```python
from build123d import *

# Parameters (mm, degrees)
SKETCH9_W                    = 200
SKETCH9_H                    = 30
BASE_FLANGE2_DEPTH           = 3
EDGE_FLANGE1_STRIP_W         = 18
EDGE_FLANGE1_STRIP_H         = 3
EDGE_FLANGE1_STRIP_CUT_DEPTH = 200
EDGE_FLANGE1_DEPTH           = 200
EDGE_FLANGE2_STRIP_W         = 18
EDGE_FLANGE2_STRIP_H         = 3
EDGE_FLANGE2_STRIP_CUT_DEPTH = 200
EDGE_FLANGE2_DEPTH           = 200
CUT_EXTRUDE1_START           = -3
CUT_EXTRUDE1_OUTLINE_R       = 4
CUT_EXTRUDE1_DEPTH           = 3
CUT_EXTRUDE1_START_2         = -100
CUT_EXTRUDE1_2_DEPTH         = 50
CUT_EXTRUDE1_START_3         = 50
CUT_EXTRUDE1_3_DEPTH         = 50
SKETCH19_R                   = 3
CUT_EXTRUDE2_DEPTH           = 3


# Read off the part's stored shape, not the designer's step: Cut-Extrude1
# Sheet-metal steps are written as plain solids
with BuildPart() as part:
    # Sketch9 → Base-Flange2 (new body)
    with BuildSketch(Plane(origin=(0, 0, 0), x_dir=(1, 0, 0), z_dir=(0, 1, 0))):
        with Locations((0, 15)):
            Rectangle(SKETCH9_W, SKETCH9_H)
    extrude(amount=-BASE_FLANGE2_DEPTH)

    # Edge-Flange1 strip (across the edge) → Edge-Flange1 strip cut (cut)
    with BuildSketch(Plane(origin=(100, -3, 0), x_dir=(0, 0, -1), z_dir=(-1, 0, 0))):
        with Locations((-6, -1.5)):
            Rectangle(EDGE_FLANGE1_STRIP_W, EDGE_FLANGE1_STRIP_H)
    extrude(amount=EDGE_FLANGE1_STRIP_CUT_DEPTH, mode=Mode.SUBTRACT)

    # Edge-Flange1 section (across the edge) → Edge-Flange1 (add)
    with BuildSketch(Plane(origin=(100, -3, 0), x_dir=(0, 0, -1), z_dir=(-1, 0, 0))):
        with BuildLine():
            Line((-3, 3), (-3, 35))
            Line((-3, 35), (0, 35))
            Line((0, 35), (0, 3))
            ThreePointArc((0, 3), (0.878679656, 0.878679656), (3, 0))
            Line((3, 0), (3, -3))
            ThreePointArc((3, -3), (-1.242640687, -1.242640687), (-3, 3))
        make_face()
    extrude(amount=EDGE_FLANGE1_DEPTH)

    # Edge-Flange2 strip (across the edge) → Edge-Flange2 strip cut (cut)
    with BuildSketch(Plane(origin=(-100, -38, 3), x_dir=(0, 1, 0), z_dir=(1, 0, 0))):
        with Locations((-6, -1.5)):
            Rectangle(EDGE_FLANGE2_STRIP_W, EDGE_FLANGE2_STRIP_H)
    extrude(amount=EDGE_FLANGE2_STRIP_CUT_DEPTH, mode=Mode.SUBTRACT)

    # Edge-Flange2 section (across the edge) → Edge-Flange2 (add)
    with BuildSketch(Plane(origin=(-100, -38, 3), x_dir=(0, 1, 0), z_dir=(1, 0, 0))):
        with BuildLine():
            Line((-3, 3), (-3, 70))
            Line((-3, 70), (0, 70))
            Line((0, 70), (0, 3))
            ThreePointArc((0, 3), (0.878679656, 0.878679656), (3, 0))
            Line((3, 0), (3, -3))
            ThreePointArc((3, -3), (-1.242640687, -1.242640687), (-3, 3))
        make_face()
    extrude(amount=EDGE_FLANGE2_DEPTH)

    # Cut-Extrude1 outline → Cut-Extrude1 (cut)
    with BuildSketch(Plane(origin=(0, -38, 0), x_dir=(1, 0, 0), z_dir=(0, 1, 0)).offset(CUT_EXTRUDE1_START)):
        with Locations((0, -25.63)):
            Circle(CUT_EXTRUDE1_OUTLINE_R)
    extrude(amount=CUT_EXTRUDE1_DEPTH, mode=Mode.SUBTRACT)

    # Cut-Extrude1 2 outline → Cut-Extrude1 2 (cut)
    with BuildSketch(Plane.YZ.offset(CUT_EXTRUDE1_START_2)):
        with BuildLine():
            ThreePointArc((-41, 6), (-40.795554958, 4.447085729), (-40.196152423, 3))
            Line((-40.196152423, 3), (-37.598076212, 4.5))
            ThreePointArc((-37.598076212, 4.5), (-37.897777479, 5.223542864), (-38, 6))
            Line((-38, 6), (-38, 73))
            Line((-38, 73), (-41, 73))
            Line((-41, 73), (-41, 6))
        make_face()
    extrude(amount=CUT_EXTRUDE1_2_DEPTH, mode=Mode.SUBTRACT)

    # Cut-Extrude1 3 outline → Cut-Extrude1 3 (cut)
    with BuildSketch(Plane.YZ.offset(CUT_EXTRUDE1_START_3)):
        with BuildLine():
            ThreePointArc((-41, 6), (-40.795554958, 4.447085729), (-40.196152423, 3))
            Line((-40.196152423, 3), (-37.598076212, 4.5))
            ThreePointArc((-37.598076212, 4.5), (-37.897777479, 5.223542864), (-38, 6))
            Line((-38, 6), (-38, 73))
            Line((-38, 73), (-41, 73))
            Line((-41, 73), (-41, 6))
        make_face()
    extrude(amount=CUT_EXTRUDE1_3_DEPTH, mode=Mode.SUBTRACT)

    # Sketch19 → Cut-Extrude2 (cut)
    with BuildSketch(Plane(origin=(0, 0, 0), x_dir=(1, 0, 0), z_dir=(0, 1, 0))):
        with Locations(Location((-90, 15, 0), (0, 0, 270))):
            Circle(SKETCH19_R)
        with Locations(Location((-50, 15, 0), (0, 0, 270))):
            Circle(SKETCH19_R)
        with Locations(Location((50, 15, 0), (0, 0, 270))):
            Circle(SKETCH19_R)
        with Locations(Location((90, 15, 0), (0, 0, 270))):
            Circle(SKETCH19_R)
    extrude(amount=-CUT_EXTRUDE2_DEPTH, mode=Mode.SUBTRACT)


solid = part.part
```
For this review, take the finished solid that the model builds, in its own axes (mm). A direction names the side the tool comes from. Give positions to 0.01 mm unless a question says otherwise; leave off trailing zeros. Write each loop counter-clockwise with the first axis right and the second up, starting at its lowest first coordinate (ties: lowest second). Pieces come first, ordered by that corner, then holes. Notation, with made-up numbers: M -29.5,38 L -3.5,38 A24 cw -3.5,61 Z; hole C 15.5,-39.5 d9. An arc over 180 degrees is marked long. One line per item, written item: value.
1) For faces 4 (the flat face through (-1, -3, -17)), 5 (the cylindrical face through (-47, -1, -15)), 6 (the flat face through (1, -20, 3)), list the 3-axis set-ups (+Z, -Z, +X, -X, +Y, -Y) from which the entire face can be reached by the end or side of a thin tool; tool diameter is ignored.
Results are:
face 4: -Z, +X, -X, -Y
face 5: +Y, -Y
face 6: +Z, +X, -X, +Y
2) Take a section at A-A, the plane z = 25.63. Write out the cut boundary in (x, y), then the cut area to 3 significant figures.
Results are:
outline: M -50,-41 L -4,-41 L -4,-38 L -50,-38 Z; M 4,-41 L 50,-41 L 50,-38 L 4,-38 Z
area: 276 mm²
3) Take a section at C-C, the plane x = -7. Write out the cut boundary in (y, z), then the cut area to 3 significant figures.
Results are:
outline: M -41,6 A6 ccw -35,0 L -6,0 A3 cw -3,-3 L -3,-30 L 0,-30 L 0,-3 A6 ccw -6,3 L -35,3 A3 cw -38,6 L -38,73 L -41,73 Z
area: 411 mm²
4) For P1, Ø8, axis at x = 50, z = -15, coming from the -Y side; P2, Ø1, axis at y = -39, z = 24, coming from the +X side; P3, Ø8.5, axis at x = 36, y = -26.5, coming from the +Z side; P4, Ø5, axis at x = -50, z = -15, coming from the -Y side, all flat-tipped, find the tip position at first contact; note any pin that passes through.
Results are:
P1: stops at y = -3
P2: stops at x = 50
P3: stops at z = 3
P4: passes through
5) For line 1 (X direction, y = -1.45, z = -15); line 2 (Z direction, x = -82, y = -32.5); line 3 (Y direction, x = -39.5, z = -12.5), list the stretches that pass through material, from the lowest coordinate up. Write a range as from..to.
Results are:
line 1: x = -100..-93, -87..-53, -47..47, 53..87, 93..100
line 2: z = 0..3
line 3: y = -3..0
6) Take a section at B-B, the plane x = 90. Write out the cut boundary in (y, z).
Results are:
outline: M -40.2,3 A6 ccw -35,0 L -6,0 A3 cw -3,-3 L -3,-12 L 0,-12 L 0,-3 A6 ccw -6,3 L -35,3 A3 cw -37.6,4.5 Z; M -3,-30 L 0,-30 L 0,-18 L -3,-18 Z
7) Take a section at D-D, the plane z = -15. Write out the cut boundary in (x, y).
Results are:
outline: M -100,-3 L -93,-3 L -93,0 L -100,0 Z; M -87,-3 L -53,-3 L -53,0 L -87,0 Z; M -47,-3 L 47,-3 L 47,0 L -47,0 Z; M 53,-3 L 87,-3 L 87,0 L 53,0 Z; M 93,-3 L 100,-3 L 100,0 L 93,0 Z
8) The part is to be moulded in two halves that separate along X. For faces 1 (the flat face through (-1, -41, 39)), 2 (the cylindrical face through (-92.93, -1.48, -15.65)), 3 (the flat face through (-100, -13, 1)), say which applies: +X half, -X half, draft (parallel to the pull), parting line (faces both ways), or undercut.
Results are:
face 1: draft
face 2: undercut
face 3: -X half
